Autodesk Inventor part; units mm, degrees
ref_plane "YZ Plane" through (0, 0, 0) normal (1, 0, 0) x (0, 1, 0)
ref_plane "XZ Plane" through (0, 0, 0) normal (0, 1, 0) x (-1, 0, 0)
ref_plane "XY Plane" through (0, 0, 0) normal (0, 0, 1) x (1, 0, 0)
sketch "Sketch1" plane through (0, 0, 0) normal (0, 0, 1) x (1, 0, 0)
  line L0 (0, 0) -> (-81.661, 0)
  line L1 (-81.661, 0) -> (-77.5429, 14.6731)
  line L2 (-77.5429, 14.6731) -> (0, 8.509)
  line L3 (0, 8.509) -> (0, 0)
  dimension "d0" = 81.661
  dimension "d1" = 15.24
  dimension "d2" = 77.7875
  dimension "d3" = 8.509
extrude "Extrusion1" add sketch "Sketch1" along normal mid plane 64.389
fillet "Fillet1" radius 1.5875 8 edges at (-38.7714, 11.591, 32.1945) (0, 8.509, 0) (0, 4.2545, 32.1945) (0, 4.2545, -32.1945) (-38.7714, 11.591, -32.1945) (-77.5429, 14.6731, 0) (-79.6019, 7.3365, -32.1945) (-79.6019, 7.3365, 32.1945)
shell "Shell1" thickness 1.905 removed faces 1 at (-53.8706, 0, 10.7315)
sketch "Sketch3" plane through (-1.4617, 8.6252, 30.607) normal (0.0792423, 0.9968554, 0) x (0.9968554, -0.0792423, 0)
  line L0 (-33.3933, 2.032) -> (-71.4933, 2.032)
  line L1 (-71.4933, 2.032) -> (-71.4933, 59.182)
  line L2 (-71.4933, 59.182) -> (-33.3933, 59.182)
  line L3 (-33.3933, 59.182) -> (-33.3933, 2.032)
  line L4 (-75.0156, 0) -> (-75.0156, 61.214)
  line L5 (-76.5733, 61.214) -> (-76.5733, 0)
  line L6 (2.1406, 30.607) -> (-92.8395, 30.607)
  point P0 (-71.4933, 30.607)
  dimension "d8" = 57.15
  dimension "d9" = 38.1
  dimension "d11" = 5.08
extrude "Extrusion2" cut sketch "Sketch3" against normal blind 0.508
fillet "Fillet2" radius 1.27 4 edges at (-34.7702, 11.0172, -28.575) (-72.7503, 14.0363, -28.575) (-72.7503, 14.0363, 28.575) (-34.7702, 11.0172, 28.575)
sketch "Sketch4" plane through (-77.8957, 13.4161, -30.607) normal (-0.9627994, 0.2702173, 0) x (0, 0, 1)
  line L0 (61.214, -13.9344) -> (0, -13.9344)
  line L1 (30.607, -13.9344) -> (30.607, -2.8384)
  point P0 (30.607, 8.1318)
  point P1 (30.607, -9.7434)
  dimension "d15" = 4.191
hole "Hole1" at (-80.5285, 4.0351, 0) direction (0.9627994, -0.2702173, 0) diameter 2.159 end through all
sketch "Sketch5" plane through (0, 0, -32.1945) normal (0, 0, -1) x (-1, 0, 0)
  line L0 (0, 7.0427) -> (0, 0)
  line L1 (1.5875, 0) -> (80.0122, 0)
  point P0 (6.35, 3.175)
  dimension "d23" = 6.35
  dimension "d24" = 3.175
hole "Hole2" at (-6.35, 3.175, -32.1945) direction (0, 0, 1) diameter 2.159 end through all
properties part number "Pedal" material "Steel, Cast"
Can you work these out from the model? Positions are in its coordinate system, mm. A direction names the side the tool comes from. Give positions to 0.01 mm unless a question says otherwise; leave off trailing zeros. Return JSON: item names as keys, results as strings.
Q1. For pin 1 Ø2.5 at (x, y) = (-53, 13) entering from +Z; pin 2 Ø1 at (y, z) = (6, -21.5) entering from -X; pin 3 Ø1.9 at (x, y) = (-6.35, 3.175) entering from -Z; pin 4 Ø12 at (x, z) = (-46.5, 21.5) entering from +Y, each with a flat end and sliding along its axis, tell me the tip position at first contact or that it passes through.
Checks:
{"pin 1": "stops at z = 32.07", "pin 2": "stops at x = -80.12", "pin 3": "passes through", "pin 4": "stops at y = 12.17"}
Q2. I need wall thicknesses on probe 1 along Z at (x, y) = (-43, 2.75); probe 2 along Z at (x, y) = (-71.5, 12.75); probe 3 along X at (y, z) = (2.75, 29) (3 decimals). Which ranges of each line are inside material? Lowest first, please.
Checks:
{"probe 1": "z = -32.19 to -30.29, 30.29 to 32.19", "probe 2": "z = -32.19 to 32.19", "probe 3": "x = -80.889 to -78.911, -1.905 to 0"}
Q3. I want a section at B-B, the plane x = -6.35. Count the separate pieces of the cut face and the enclosed holes in it, then the cut area to 3 significant figures.
Checks:
{"separate pieces": "3", "enclosed holes": "0", "area": "141 mm2"}
Q4. We'd pull the mould along Y, two halves only. Please class faces 3 (the face through (-77.29, 14.28, -0.43)), 4 (the face through (-79.69, 3.46, 1.03)), 5 (the face through (0, 4, 0)), 6 (the face through (-39.54, 9.74, -0.42)): released by +Y, released by -Y, zero draft, split by the parting line, or undercut.
Checks:
{"face 3": "released by +Y", "face 4": "undercut", "face 5": "zero draft", "face 6": "released by -Y"}
Q5. On a 3-axis mill with a long thin cutter (end or side, diameter ignored), from which of +Z, -Z, +X, -X, +Y, -Y can I reach the whole of each face in a straight line? I mean faces 1 (the face through (-78, 6, 0)), 2 (the face through (-14.448, 9.658, -0.428)). Say none if no direction works.
Checks:
{"face 1": "-Y", "face 2": "+Z, -Z, +X, +Y"}
